from build123d import *

# Parameters (mm, degrees)
BOSS_EXTRUDE1_DEPTH    = 381
F_10_32_TAPPED_HOLE5_D = 4.0386
F_10_32_TAPPED_HOLE6_D = 4.0386


with BuildPart() as part:
    # Sketch1 → Boss-Extrude1 (new body)
    with BuildSketch(Plane.XY):
        Polygon((0, 0), (0, 50.8), (6.35, 50.8), (6.35, 6.35), (35.56, 6.35), (35.56, 0), align=None)
    extrude(amount=BOSS_EXTRUDE1_DEPTH)

    # #10-32 Tapped Hole5 (through all)
    with Locations(Plane(origin=(6.35, 0, 0), x_dir=(0, 0, -1), z_dir=(1, 0, 0))):
        with Locations((-355.6, 25.4), (-25.4, 25.4)):
            Hole(F_10_32_TAPPED_HOLE5_D / 2)

    # #10-32 Tapped Hole6 (through all)
    with Locations(Plane(origin=(0, 6.35, 0), x_dir=(-1, 0, 0), z_dir=(0, 1, 0))):
        with Locations((-27.94, 356.095307591), (-27.94, 25.895307591)):
            Hole(F_10_32_TAPPED_HOLE6_D / 2)


solid = part.part
Input: part model. Units: mm. Frame: model coordinates. A direction names the side the tool comes from. Coordinates: 2 decimals unless noted, no trailing zeros. Order: outer loops, then holes, each group sorted by start corner. A loop starts at its lowest first (then second) coordinate and runs counter-clockwise, first axis right, second up.
1. Contact query for flat-ended pins moving along their axis: P1, Ø6.5, axis at y = 25.4, z = 25.4, coming from the +X side; P2, Ø8, axis at x = 25.5, z = 55, coming from the +Y side. Output: stop coordinate, or through.
Checked values:
P1: stops at x = 6.35
P2: stops at y = 6.35
2. Ray query, line 1 along Z through (x, y) = (27.94, 4.75); line 2 along X through (y, z) = (27.5, 63.5). Return the intervals inside material, ascending.
Checked values:
line 1: z = 0 to 23.88, 27.91 to 354.08, 358.11 to 381
line 2: x = 0 to 6.35
3. Cut plane A-A, the plane z = 156. Return loops of the section in (x, y).
Checked values:
outline: (0, 0) - (35.56, 0) - (35.56, 6.35) - (6.35, 6.35) - (6.35, 50.8) - (0, 50.8) - close
4. Access query for faces 1 (the flat face through (3, 50.8, 188)), 2 (the flat face through (21, 6.35, 188)). Directions: +Z, -Z, +X, -X, +Y, -Y. A direction counts if a zero-diameter tool reaches every point of the face in a straight line with its end or side. Return the directions, or none.
Checked values:
face 1: +Z, -Z, +X, -X, +Y
face 2: +Z, -Z, +X, +Y
5. Cut plane B-B, the plane y = 10. Return loops of the section in (x, z), plus the area to 3 significant figures.
Checked values:
outline: (0, 0) - (6.35, 0) - (6.35, 381) - (0, 381) - close
area: 2,420 mm2
